Check sheet for the modelled part. Datum: model origin and axes. Units: mm. Face numbers are marked on the shaded views. A direction names the side the tool comes from. Round coordinates to 2 decimals unless told otherwise and drop trailing zeros. Write each loop counter-clockwise with the first axis right and the second up, starting at its lowest first coordinate (ties: lowest second). Pieces come first, ordered by that corner, then holes. Notation, with made-up numbers: (-23, -39) - (20, -39) arc R27 ccw to (20, -3) - close; hole circle Ø11 at (-32, 26). An arc over 180 degrees is marked (long way). Use one line per item in the form item = value. Start each with the question number.
1) Set-up check for the marked faces 1 and 2: record each of +Z, -Z, +X, -X, +Y, -Y from which the full face is reachable in a straight line by a thin tool's end or side.
2) Section check A-A (y = 4). Record the boundary of the cut face in (x, z).
3) Section check B-B (y = 5.5). Record the boundary of the cut face in (x, z) (1 decimal), then the cut area to 3 significant figures.
4) Section check C-C (y = 1.5). Record the boundary of the cut face in (x, z) (1 decimal).
5) Scan lines: probe 1 along Z at (x, y) = (0.25, 3); probe 2 along Y at (x, z) = (-1.25, -2); probe 3 along Z at (x, y) = (-2, 4.5). Record each from-to range of solid material in increasing order.
6) Gauge pin test, flat ends, axial feed: P1, Ø3, axis at x = -2.5, y = 2, coming from the +Z side; P2, Ø3, axis at x = 2, y = 2, coming from the -Z side; P3, Ø4, axis at x = 2.5, y = 8.5, coming from the -Z side. Record the tip position at first contact, or that the pin passes through.
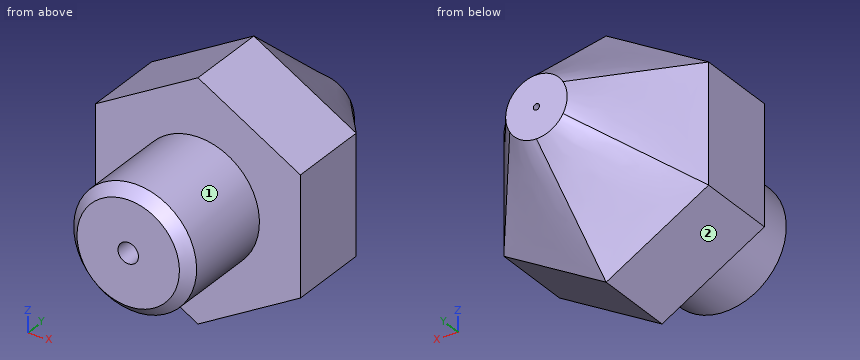
from build123d import *

# Parameters (mm, degrees)
SKETCH1_R           = 3
BOSS_EXTRUDE1_DEPTH = 5
BOSS_EXTRUDE2_DEPTH = 4
CHAMFER1_SIZE       = 0.5
SKETCH5_R           = 0.15
SKETCH4_R           = 0.5


with BuildPart() as part:
    # Sketch1 → Boss-Extrude1 (new body)
    with BuildSketch(Plane(origin=(0, 0, 0), x_dir=(1, 0, 0), z_dir=(0, 1, 0))):
        with Locations(Location((0, 0, 0), (0, 0, 270))):
            Circle(SKETCH1_R)
    extrude(amount=BOSS_EXTRUDE1_DEPTH)

    # Sketch2 → Boss-Extrude2 (add)
    with BuildSketch(Plane(origin=(0, 5, 0), x_dir=(1, 0, 0), z_dir=(0, 1, 0))):
        Polygon((0, 5.773502692), (-5, 2.886751346), (-5, -2.886751346), (0, -5.773502692), (5, -2.886751346), (5, 2.886751346), align=None)
    extrude(amount=BOSS_EXTRUDE2_DEPTH)

    # Chamfer1
    chamfer1_edges = [part.edges().sort_by_distance(p)[0] for p in [
        (0, 0, -3),
    ]]
    chamfer(chamfer1_edges, length=CHAMFER1_SIZE)

    # Loft1: read off the stored shape, not the designer's step
    # Loft1: loft between two sections, ruled curve by curve
    loft1_from = [
        Edge.make_bspline([(1.299038106, 14, -0.75), (1.424038106, 14, -0.533493649), (1.5, 14, -0.267949192), (1.5, 14, 0.267949192), (1.424038106, 14, 0.533493649), (1.299038106, 14, 0.75)], [0, 0, 0, 0, 0.5, 0.5, 1, 1, 1, 1], 3),
        Edge.make_bspline([(1.299038106, 14, 0.75), (1.174038106, 14, 0.966506351), (0.982050808, 14, 1.165063509), (0.517949192, 14, 1.433012702), (0.25, 14, 1.5), (0, 14, 1.5)], [0, 0, 0, 0, 0.5, 0.5, 1, 1, 1, 1], 3),
        Edge.make_bspline([(0, 14, -1.5), (0.25, 14, -1.5), (0.517949192, 14, -1.433012702), (0.982050808, 14, -1.165063509), (1.174038106, 14, -0.966506351), (1.299038106, 14, -0.75)], [0, 0, 0, 0, 0.5, 0.5, 1, 1, 1, 1], 3),
        Edge.make_bspline([(0, 14, 1.5), (-0.25, 14, 1.5), (-0.517949192, 14, 1.433012702), (-0.982050808, 14, 1.165063509), (-1.174038106, 14, 0.966506351), (-1.299038106, 14, 0.75)], [0, 0, 0, 0, 0.5, 0.5, 1, 1, 1, 1], 3),
        Edge.make_bspline([(-1.299038106, 14, 0.75), (-1.424038106, 14, 0.533493649), (-1.5, 14, 0.267949192), (-1.5, 14, -0.267949192), (-1.424038106, 14, -0.533493649), (-1.299038106, 14, -0.75)], [0, 0, 0, 0, 0.5, 0.5, 1, 1, 1, 1], 3),
        Edge.make_bspline([(-1.299038106, 14, -0.75), (-1.174038106, 14, -0.966506351), (-0.982050808, 14, -1.165063509), (-0.517949192, 14, -1.433012702), (-0.25, 14, -1.5), (0, 14, -1.5)], [0, 0, 0, 0, 0.5, 0.5, 1, 1, 1, 1], 3),
    ]
    loft1_to = [
        Edge.make_bspline([(5, 9, -2.886751346), (5, 9, -1.924500897), (5, 9, -0.962250449), (5, 9, 0.962250449), (5, 9, 1.924500897), (5, 9, 2.886751346)], [0, 0, 0, 0, 0.5, 0.5, 1, 1, 1, 1], 3),
        Edge.make_bspline([(5, 9, 2.886751346), (4.166666667, 9, 3.36787657), (3.333333333, 9, 3.849001795), (1.666666667, 9, 4.811252243), (0.833333333, 9, 5.292377468), (0, 9, 5.773502692)], [0, 0, 0, 0, 0.5, 0.5, 1, 1, 1, 1], 3),
        Edge.make_bspline([(0, 9, -5.773502692), (0.833333333, 9, -5.292377468), (1.666666667, 9, -4.811252243), (3.333333333, 9, -3.849001795), (4.166666667, 9, -3.36787657), (5, 9, -2.886751346)], [0, 0, 0, 0, 0.5, 0.5, 1, 1, 1, 1], 3),
        Edge.make_bspline([(0, 9, 5.773502692), (-0.833333333, 9, 5.292377468), (-1.666666667, 9, 4.811252243), (-3.333333333, 9, 3.849001795), (-4.166666667, 9, 3.36787657), (-5, 9, 2.886751346)], [0, 0, 0, 0, 0.5, 0.5, 1, 1, 1, 1], 3),
        Edge.make_bspline([(-5, 9, 2.886751346), (-5, 9, 1.924500897), (-5, 9, 0.962250449), (-5, 9, -0.962250449), (-5, 9, -1.924500897), (-5, 9, -2.886751346)], [0, 0, 0, 0, 0.5, 0.5, 1, 1, 1, 1], 3),
        Edge.make_bspline([(-5, 9, -2.886751346), (-4.166666667, 9, -3.36787657), (-3.333333333, 9, -3.849001795), (-1.666666667, 9, -4.811252243), (-0.833333333, 9, -5.292377468), (0, 9, -5.773502692)], [0, 0, 0, 0, 0.5, 0.5, 1, 1, 1, 1], 3),
    ]
    loft1 = Solid(Shell([*[Face.make_surface_from_curves(loft1_from[k], loft1_to[k]) for k in range(6)], Face(Wire(loft1_from)), Face(Wire(loft1_to))]))
    add(loft1)

    # Sketch5 → Cut-Loft1 section 0
    with BuildSketch(Plane(origin=(0, 14, 0), x_dir=(-1, 0, 0), z_dir=(0, 1, 0))):
        Circle(SKETCH5_R)
    # Sketch4 → Cut-Loft1 section 1
    with BuildSketch(Plane.XZ):
        Circle(SKETCH4_R)
    loft(mode=Mode.SUBTRACT)


solid = part.part
Results are:
q1.face_1 = -Y
q1.face_2 = -Z, -X, +Y, -Y
q2.outline = circle Ø6 at (0, 0); hole circle Ø0.8 at (0, 0)
q3.outline = (-5, -2.9) - (0, -5.8) - (5, -2.9) - (5, 2.9) - (0, 5.8) - (-5, 2.9) - close; hole circle Ø0.7 at (0, 0)
q3.area = 86.2 mm²
q4.outline = circle Ø6 at (0, 0); hole circle Ø0.9 at (0, 0)
q5.probe_1 = -2.99 to -0.34, 0.34 to 2.99
q5.probe_2 = 0 to 12.77
q5.probe_3 = -2.24 to 2.24
q6.P1 = 2.83
q6.P2 = -2.96
q6.P3 = -5.48
